The listing builds one solid part. Answer for the finished solid, in the listing's coordinates (mm). A direction names the side the tool comes from. Coordinates: 2 decimals unless noted, no trailing zeros. Order: outer loops, then holes, each group sorted by start corner. A loop starts at its lowest first (then second) coordinate and runs counter-clockwise, first axis right, second up.
```python
from build123d import *


with BuildPart() as part:
    # Sketch1 → Revolve1 (revolve)
    with BuildSketch(Plane(origin=(0, 0, 0), x_dir=(0, 0, -1), z_dir=(1, 0, 0))):
        with BuildLine():
            Line((-15, 14), (-15, 12))
            Line((-15, 12), (-14, 12))
            ThreePointArc((-14, 12), (-15.496575182, 6.08276253), (-16, 0))
            Line((-16, 0), (18.1, 0))
            Line((18.1, 0), (18.1, 12.75))
            Line((18.1, 12.75), (12, 12.75))
            Line((12, 12.75), (12, 14.5))
            Line((12, 14.5), (-15, 14.5))
            Line((-15, 14.5), (-15, 14))
        make_face()
    revolve(axis=Axis((0, 0, -18.1), (0, 0, 1)))


solid = part.part
```
(1) Find section C-C (z = 4). Write down the section's boundary in (x, y).
(2) For faces 4 (the face through (12.864, 6.691, 1.689)), 5 (the face through (-12, 2, 15)), determine the directions among +Z, -Z, +X, -X, +Y, -Y from which every point of the face is accessible in a straight line to the end or side of a thin tool.
(3) Consider line 1 (Z direction, x = 7.75, y = -10.25); line 2 (Z direction, x = -11.5, y = 3.75); line 3 (X direction, y = 4.25, z = -14). Determine where each line is inside the solid, lowest interval first.
(4) Each of these flat-tipped pins is pushed along its axis until it touches: pin 1 Ø1 at (x, z) = (-8.5, -10) entering from -Y; pin 2 Ø1 at (x, y) = (2, 11.5) entering from +Z; pin 3 Ø3 at (y, z) = (-9.5, -1.5) entering from -X. Where does it stop, or does it pass through?
(5) Find section A-A (x = 0). Write down the section's boundary in (y, z).
(6) The mould has two halves that part along Y. Classify faces 1 (the face through (13, 0, -12)), 2 (the face through (12.447, -2.764, -15.007)), 3 (the face through (-0.53, -11.99, 14.49)): released by +Y, released by -Y, zero draft, split by the parting line, or undercut.
(7) Find section D-D (y = -7.75). Write down the section's boundary in (x, z).
Findings below:
1. outline: circle Ø29 at (0, 0)
2. face 4: +Z, -Z
2. face 5: +Z
3. line 1: z = -12 to 15
3. line 2: z = -18.1 to 15
3. line 3: x = -12.02 to 12.02
4. pin 1: stops at y = -12.09
4. pin 2: stops at z = 15
4. pin 3: stops at x = -12.09
5. outline: (-14.5, -12) - (-12.75, -12) - (-12.75, -18.1) - (12.75, -18.1) - (12.75, -12) - (14.5, -12) - (14.5, 15) - (12, 15) - (12, 14) arc R37 ccw to (-12, 14) - (-12, 15) - (-14.5, 15) - close
6. face 1: zero draft
6. face 2: split by the parting line
6. face 3: undercut
7. outline: (-12.26, -12) - (-10.12, -12) - (-10.12, -18.1) - (10.12, -18.1) - (10.12, -12) - (12.26, -12) - (12.26, 15) - (9.16, 15) - (9.16, 14) arc R36.18 ccw to (-9.16, 14) - (-9.16, 15) - (-12.26, 15) - close
